from build123d import *

# Parameters (mm, degrees)
SKETCH1_W           = 22.5
SKETCH1_H           = 11.8
BOSS_EXTRUDE1_DEPTH = 26.7
SKETCH2_W           = 2.5
SKETCH2_H           = 11.8
BOSS_EXTRUDE2_DEPTH = 4.7
SKETCH5_W           = 2.5
SKETCH5_H           = 11.8
BOSS_EXTRUDE3_DEPTH = 4.7
CUT_EXTRUDE1_DEPTH  = 6.2
FILLET1_R           = 2.5
FILLET2_R           = 2.5
CUT_EXTRUDE2_DEPTH  = 3.2
SKETCH7_R           = 2.3
SKETCH7_R_2         = 0.85
BOSS_EXTRUDE4_DEPTH = 3.2
CUT_EXTRUDE3_DEPTH  = 2.5
CUT_EXTRUDE4_DEPTH  = 2.5


with BuildPart() as part:
    # Sketch1 → Boss-Extrude1 (new body)
    with BuildSketch(Plane.XY):
        with Locations((3.150909091, 4.478636364)):
            Rectangle(SKETCH1_W, SKETCH1_H)
    extrude(amount=BOSS_EXTRUDE1_DEPTH)

    # Sketch2 → Boss-Extrude2 (add)
    with BuildSketch(Plane(origin=(14.400909091, 0, 0), x_dir=(0, 0, -1), z_dir=(1, 0, 0))):
        with Locations((-17.25, 4.478636364)):
            Rectangle(SKETCH2_W, SKETCH2_H)
    extrude(amount=BOSS_EXTRUDE2_DEPTH)

    # Sketch5 → Boss-Extrude3 (add)
    with BuildSketch(Plane.ZY.offset(8.099090909)):
        with Locations((17.15, 4.478636364)):
            Rectangle(SKETCH5_W, SKETCH5_H)
    extrude(amount=BOSS_EXTRUDE3_DEPTH)

    # Sketch6 → Cut-Extrude1 (cut)
    with BuildSketch(Plane.XY.offset(26.7)):
        with BuildLine():
            Line((5.800909091, 1.978636364), (3.145064777, 1.978636364))
            ThreePointArc((3.145064777, 1.978636364), (0.967926621, -0.499315019), (-2.199090896, -1.421363636))
            Line((-2.199090896, -1.421363636), (14.400909091, -1.421363636))
            Line((14.400909091, -1.421363636), (14.400909091, 10.378636364))
            Line((14.400909091, 10.378636364), (-2.199090917, 10.378636364))
            ThreePointArc((-2.199090917, 10.378636364), (0.967926612, 9.456587752), (3.145064777, 6.978636364))
            Line((3.145064777, 6.978636364), (5.800909091, 6.978636364))
            Line((5.800909091, 6.978636364), (5.800909091, 1.978636364))
        make_face()
        with BuildLine():
            Line((-8.099090909, -1.421363636), (-2.199090896, -1.421363636))
            ThreePointArc((-2.199090896, -1.421363636), (-6.371020914, 0.30670635), (-8.099090909, 4.478636364))
            Line((-8.099090909, 4.478636364), (-8.099090909, -1.421363636))
        make_face()
        with BuildLine():
            Line((-8.099090909, 10.378636364), (-8.099090909, 4.478636364))
            ThreePointArc((-8.099090909, 4.478636364), (-6.371020921, 8.65056637), (-2.199090917, 10.378636364))
            Line((-2.199090917, 10.378636364), (-8.099090909, 10.378636364))
        make_face()
    extrude(amount=-CUT_EXTRUDE1_DEPTH, mode=Mode.SUBTRACT)

    # Fillet1
    fillet1_edges = [part.edges().sort_by_distance(p)[0] for p in [
        (5.800909091, 1.978636364, 23.6),
    ]]
    fillet(fillet1_edges, radius=FILLET1_R)

    # Fillet2
    fillet2_edges = [part.edges().sort_by_distance(p)[0] for p in [
        (5.800909091, 6.978636364, 23.6),
    ]]
    fillet(fillet2_edges, radius=FILLET2_R - 0.0001)  # a hair under: the kernel refuses the full size

    # Sketch6<3> → Cut-Extrude2 (cut)
    with BuildSketch(Plane.XY.offset(26.7)):
        with BuildLine():
            Line((3.145064777, 1.978636364), (5.800909091, 1.978636364))
            Line((5.800909091, 1.978636364), (5.800909091, 6.978636364))
            Line((5.800909091, 6.978636364), (3.145064777, 6.978636364))
            ThreePointArc((3.145064777, 6.978636364), (-8.099090909, 4.478636364), (3.145064777, 1.978636364))
        make_face()
    extrude(amount=-CUT_EXTRUDE2_DEPTH, mode=Mode.SUBTRACT)

    # Sketch7 → Boss-Extrude4 (add)
    with BuildSketch(Plane.XY.offset(23.5)):
        with Locations((-2.199090909, 4.478636364)):
            Circle(SKETCH7_R)
        with Locations((-2.199090909, 4.478636364)):
            Circle(SKETCH7_R_2, mode=Mode.SUBTRACT)
    extrude(amount=BOSS_EXTRUDE4_DEPTH)

    # Sketch11 → Cut-Extrude3 (cut)
    with BuildSketch(Plane.XY.offset(18.4)):
        with BuildLine():
            Line((-12.865758951, 3.828636364), (-11.259025117, 3.828636364))
            ThreePointArc((-11.259025117, 3.828636364), (-9.499090909, 4.478636364), (-11.259025117, 5.128636364))
            Line((-11.259025117, 5.128636364), (-12.865758951, 5.128636364))
            Line((-12.865758951, 5.128636364), (-12.865758951, 3.828636364))
        make_face()
    extrude(amount=-CUT_EXTRUDE3_DEPTH, mode=Mode.SUBTRACT)

    # Sketch12 → Cut-Extrude4 (cut)
    with BuildSketch(Plane.XY.offset(18.5)):
        with BuildLine():
            Line((17.560843299, 3.828636364), (19.100909091, 3.828636364))
            Line((19.100909091, 3.828636364), (19.100909091, 5.128636364))
            Line((19.100909091, 5.128636364), (17.560843299, 5.128636364))
            ThreePointArc((17.560843299, 5.128636364), (15.800909091, 4.478636364), (17.560843299, 3.828636364))
        make_face()
    extrude(amount=-CUT_EXTRUDE4_DEPTH, mode=Mode.SUBTRACT)


solid = part.part
Design review of the part built by this model. Coordinates are the model's own, in mm. A direction names the side the tool comes from. Give positions to 0.01 mm unless a question says otherwise; leave off trailing zeros. Loops run counter-clockwise (first coordinate to the right, second up) from the corner with the lowest first, then second, coordinate; pieces in that order, holes last. Notation, with made-up numbers: (-18.75, -8) - (0.25, -8) arc R6 cw to (0.25, 0) - close; hole circle Ø8 at (-32, 12.25). An arc over 180 degrees is marked (long way). Use CSV: the item, a comma, the result in double quotes. Start each with the question number.
1. Wall thickness on L1, parallel to Z at x = -4, y = 0; L2, parallel to Z at x = 12, y = 10.25; L3, parallel to X at y = 5, z = 3.75: over which ranges is each line inside the solid? List them lowest first.
2. Draft analysis for pull direction Y (two halves, no side actions). For faces 5 (the flat face through (3, 10.379, 10)), 6 (the flat face through (-12.799, 1, 17)), 7 (the flat face through (18, 3.829, 17)), 8 (the cylindrical face through (-3.894, 6.033, 25.078)), state which applies: released by +Y, released by -Y, zero draft, split by the parting line, or undercut.
3. Add section B-B (x = 17). State the section outline as (y, z) points.
4. Add section D-D (x = -5.5). State the section outline as (y, z) points, plus the area to 3 significant figures.
5. Add section C-C (y = -0.25). State the section outline as (x, z) points, plus the area to 3 significant figures.
6. Machinability: for faces 1 (the flat face through (17, 6, 16)), 2 (the flat face through (18, 5.129, 17)), 3 (the flat face through (14.401, 4, 19)), 4 (the flat face through (-12, 5.129, 17)), which of the approach directions +Z, -Z, +X, -X, +Y, -Y give a long, thin tool a straight path to every point of the face, cutting with its end or side? Answer none if there is none.
7. Insertion check: P1, Ø2.5, axis at x = -10.5, y = 4.48, coming from the +Z side; P2, Ø2, axis at x = 1, y = 8.5, coming from the +Z side; P3, Ø2, axis at x = -8.5, z = 23, coming from the +Y side. Each pin has a flat end and moves straight along its axis. Give the tip position at first contact, or say it passes through.
Results found:
1,L1,"z = 0 to 23.5"
1,L2,"z = 0 to 20.5"
1,L3,"x = -8.1 to 14.4"
2,face 5,"released by +Y"
2,face 6,"zero draft"
2,face 7,"undercut"
2,face 8,"split by the parting line"
3,outline,"(-1.42, 16) - (3.5, 16) - (3.5, 18.5) - (-1.42, 18.5) - close; (5.46, 16) - (10.38, 16) - (10.38, 18.5) - (5.46, 18.5) - close"
4,outline,"(-1.42, 0) - (10.38, 0) - (10.38, 20.5) - (9.37, 20.5) - (9.37, 23.5) - (-0.41, 23.5) - (-0.41, 20.5) - (-1.42, 20.5) - close"
4,area,"271 mm²"
5,outline,"(-12.8, 15.9) - (-8.1, 15.9) - (-8.1, 0) - (14.4, 0) - (14.4, 16) - (19.1, 16) - (19.1, 18.5) - (14.4, 18.5) - (14.4, 20.5) - (1.33, 20.5) - (1.33, 23.5) - (-5.73, 23.5) - (-5.73, 20.5) - (-8.1, 20.5) - (-8.1, 18.4) - (-12.8, 18.4) - close"
5,area,"506 mm²"
6,face 1,"-Z, +X, +Y, -Y"
6,face 2,"+Z, -Z, +X"
6,face 3,"+Z, +X, +Y, -Y"
6,face 4,"+Z, -Z, -X"
7,P1,"stops at z = 18.4"
7,P2,"stops at z = 23.5"
7,P3,"stops at y = 7.07"
